The drawing under review shows one solid part. Ordinate dimensions are in mm from its lowest x, y, z. Coordinates: 2 decimals unless noted, no trailing zeros. Order: outer loops, then holes, each group sorted by start corner. A loop starts at its lowest first (then second) coordinate and runs counter-clockwise, first axis right, second up.
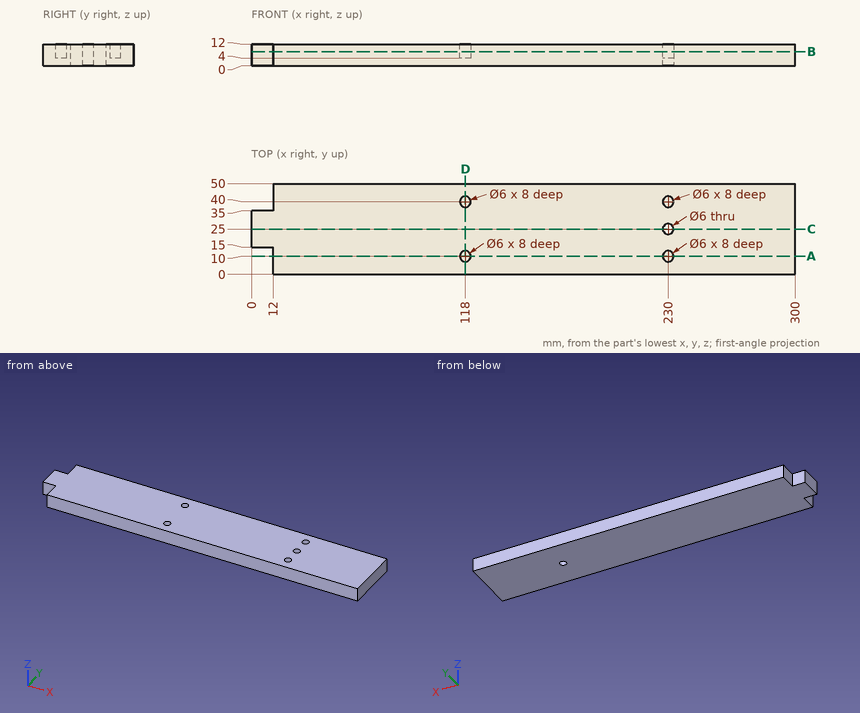
(1) We need section D-D, the plane x = 118. Write out the cut boundary in (y, z).
A:
outline: (0, 0) - (50, 0) - (50, 12) - (43, 12) - (43, 4) - (37, 4) - (37, 12) - (13, 12) - (13, 4) - (7, 4) - (7, 12) - (0, 12) - close
(2) We need section A-A, the plane y = 10. Write out the cut boundary in (x, z), and give its area (3 significant figures).
A:
outline: (12, 0) - (300, 0) - (300, 12) - (233, 12) - (233, 4) - (227, 4) - (227, 12) - (121, 12) - (121, 4) - (115, 4) - (115, 12) - (12, 12) - close
area: 3,360 mm2
(3) Wall thickness on probe 1 along Y at (x, z) = (230, 5.75); probe 2 along Y at (x, z) = (230, 3.5); probe 3 along X at (y, z) = (12.5, 8.75): over which ranges is each line inside the solid? List them lowest first.
A:
probe 1: y = 0 to 7, 13 to 22, 28 to 37, 43 to 50
probe 2: y = 0 to 22, 28 to 50
probe 3: x = 12 to 116.34, 119.66 to 228.34, 231.66 to 300
(4) We need section B-B, the plane z = 7.75. Write out the cut boundary in (x, y), and give its area (3 significant figures).
A:
outline: (0, 15) - (12, 15) - (12, 0) - (300, 0) - (300, 50) - (12, 50) - (12, 35) - (0, 35) - close; hole circle Ø6 at (118, 10); hole circle Ø6 at (118, 40); hole circle Ø6 at (230, 10); hole circle Ø6 at (230, 25); hole circle Ø6 at (230, 40)
area: 14,500 mm2
(5) We need section C-C, the plane y = 25. Write out the cut boundary in (x, z).
A:
outline: (0, 0) - (227, 0) - (227, 12) - (0, 12) - close; (233, 0) - (300, 0) - (300, 12) - (233, 12) - close
(6) For pin 1 Ø1.8 at (x, y) = (117, 41.5) entering from +Z; pin 2 Ø6 at (y, z) = (10, 7) entering from -X, all flat-tipped, find the tip position at first contact; note any pin that passes through.
A:
pin 1: stops at z = 4
pin 2: stops at x = 12
